Geometry check sheet. Reference: the model listing, model coordinates, mm. Give positions to 0.01 mm unless a question says otherwise; leave off trailing zeros. Write each loop counter-clockwise with the first axis right and the second up, starting at its lowest first coordinate (ties: lowest second). Pieces come first, ordered by that corner, then holes. Notation, with made-up numbers: (76.25, 21.5) -> (115.25, 21.5) arc R16 cw to (115.25, 45.5) -> close; hole circle Ø8 at (66.5, 34). An arc over 180 degrees is marked (long way). One line per item, written item: value.
from build123d import *

# Parameters (mm, degrees)
SKETCH_1_W      = 10
SKETCH_1_H      = 20
EXTRUDE_1_DEPTH = 50
CHAMFER_1_SIZE  = 15
CHAMFER_1_SIZE2 = 6.994614872
CHAMFER_2_SIZE  = 15
CHAMFER_2_SIZE2 = 6.994614872


with BuildPart() as part:
    # Эскиз1 → Вытянуть1 (new body)
    with BuildSketch(Plane(origin=(0, 0, 0), x_dir=(1, 0, 0), z_dir=(0, 1, 0))):
        Rectangle(SKETCH_1_W, SKETCH_1_H)
    extrude(amount=EXTRUDE_1_DEPTH)

    # Фаска1
    chamfer_1_edges = [part.edges().sort_by_distance(p)[0] for p in [
        (0, 50, 10),
    ]]
    chamfer_1_side = [part.faces().sort_by_distance(p)[0] for p in [
        (0, 25, 10),
    ]]
    chamfer(chamfer_1_edges, length=CHAMFER_1_SIZE, length2=CHAMFER_1_SIZE2, reference=chamfer_1_side[0])

    # Фаска2
    chamfer_2_edges = [part.edges().sort_by_distance(p)[0] for p in [
        (0, 50, -10),
    ]]
    chamfer_2_side = [part.faces().sort_by_distance(p)[0] for p in [
        (0, 25, -10),
    ]]
    chamfer(chamfer_2_edges, length=CHAMFER_2_SIZE, length2=CHAMFER_2_SIZE2, reference=chamfer_2_side[0])


solid = part.part
1) Sectioned sample at A-A on x = 2. Record the cut outline in (y, z), plus the area to 3 significant figures.
Verdict:
outline: (0, -10) -> (35, -10) -> (50, -3.01) -> (50, 3.01) -> (35, 10) -> (0, 10) -> close
area: 895 mm^2
2) Scan lines: probe 1 along Y at (x, z) = (3.5, 3.5); probe 2 along Z at (x, y) = (2, 43); probe 3 along Y at (x, z) = (-4, -8.75). Record each from-to range of solid material in increasing order.
Verdict:
probe 1: 0 to 48.94
probe 2: -6.27 to 6.27
probe 3: 0 to 37.68
3) Sectioned sample at C-C on y = 40. Record the cut outline in (x, z).
Verdict:
outline: (-5, -7.67) -> (5, -7.67) -> (5, 7.67) -> (-5, 7.67) -> close
4) Sectioned sample at B-B on z = 5.5. Record the cut outline in (x, y), plus the area to 3 significant figures.
Verdict:
outline: (-5, 0) -> (5, 0) -> (5, 44.65) -> (-5, 44.65) -> close
area: 447 mm^2
5) Depth check by flat-ended pin: pin 1 Ø3 at (x, z) = (1, -6) entering from +Y; pin 2 Ø6 at (x, y) = (-1.5, 38.5) entering from +Z. Enter the tip coordinate at first touch or a pass-through.
Verdict:
pin 1: y = 46.79
pin 2: z = 9.77
